from build123d import *

# Parameters (mm, degrees)
SKETCH_1_R               = 16.5
EXTRUDE_1_DEPTH          = 8
CUT_EXTRUDE_1_DEPTH      = 25.667792767
CUT_EXTRUDE_1_DEPTH_BACK = 25.667792767
SKETCH_4_R               = 2.5
SKETCH_4_R_2             = 1.9
SKETCH_1_3_R             = 10
EXTRUDE_2_DEPTH          = 8
SKETCH_1_4_R             = 10
EXTRUDE_3_DEPTH          = 60
EXTRUDE_START            = 14
SKETCH_5_R               = 16.5
EXTRUDE_4_DEPTH          = 14
CUT_EXTRUDE_START        = -14
SKETCH_6_R               = 2.5
SKETCH_6_R_2             = 1.9
CUT_EXTRUDE_2_DEPTH      = 14


with BuildPart() as part:
    # Sketch 1 → Extrude 1 (new body)
    with BuildSketch(Plane(origin=(0, 0, 0), x_dir=(1, 0, 0), z_dir=(0, 1, 0))):
        with Locations(Location((0, 0, 0), (0, 0, 270))):
            Circle(SKETCH_1_R)
    extrude(amount=EXTRUDE_1_DEPTH)

    # Sketch 4 → Cut-Extrude 1 (cut, two sides: drawn at the far end of the back side and taken through both)
    with BuildSketch(Plane(origin=(0, 8, 0), x_dir=(1, 0, 0), z_dir=(0, 1, 0)).offset(-CUT_EXTRUDE_1_DEPTH_BACK)):
        with Locations(Location((0, 10.2, 0), (0, 0, 270))):
            Circle(SKETCH_4_R)
        with Locations(Location((-6.25, 10.825317547, 0), (0, 0, 270))):
            Circle(SKETCH_4_R_2)
        with Locations(Location((6.25, 10.825317547, 0), (0, 0, 270))):
            Circle(SKETCH_4_R_2)
        with Locations(Location((12.5, 0, 0), (0, 0, 270))):
            Circle(SKETCH_4_R_2)
        with Locations(Location((6.25, -10.825317547, 0), (0, 0, 270))):
            Circle(SKETCH_4_R_2)
        with Locations(Location((-6.25, -10.825317547, 0), (0, 0, 270))):
            Circle(SKETCH_4_R_2)
        with Locations(Location((-12.5, 0, 0), (0, 0, 270))):
            Circle(SKETCH_4_R_2)
        with Locations(Location((8.833459119, -5.1, 0), (0, 0, 270))):
            Circle(SKETCH_4_R)
        with Locations(Location((-8.833459119, -5.1, 0), (0, 0, 270))):
            Circle(SKETCH_4_R)
    extrude(amount=CUT_EXTRUDE_1_DEPTH + CUT_EXTRUDE_1_DEPTH_BACK, mode=Mode.SUBTRACT)

    # Sketch 1_3 → Extrude 2 (add)
    with BuildSketch(Plane(origin=(0, 0, 0), x_dir=(1, 0, 0), z_dir=(0, 1, 0))):
        with BuildLine():
            ThreePointArc((0.989109801, 16.470326706), (16.5, 0), (0.989109801, -16.470326706))
            Line((0.989109801, -16.470326706), (100, -13.5))
            ThreePointArc((100, -13.5), (113.5, 0), (100, 13.5))
            Line((100, 13.5), (0.989109801, 16.470326706))
        make_face()
        with Locations(Location((100, 0, 0), (0, 0, 270))):
            Circle(SKETCH_1_3_R, mode=Mode.SUBTRACT)
    extrude(amount=EXTRUDE_2_DEPTH)

    # Sketch 1_4 → Extrude 3 (add)
    with BuildSketch(Plane(origin=(0, 0, 0), x_dir=(1, 0, 0), z_dir=(0, 1, 0))):
        with Locations(Location((100, 0, 0), (0, 0, 270))):
            Circle(SKETCH_1_4_R)
    extrude(amount=EXTRUDE_3_DEPTH)

    # Sketch 5 → Extrude 4 (add)
    with BuildSketch(Plane.XZ.offset(EXTRUDE_START)):
        with Locations(Location((0, 0, 0), (0, 0, 270))):
            Circle(SKETCH_5_R)
    extrude(amount=-EXTRUDE_4_DEPTH)

    # Sketch 6 → Cut-Extrude 2 (cut)
    with BuildSketch(Plane.XZ.offset(14).offset(CUT_EXTRUDE_START)):
        with Locations(Location((-8.833459119, 5.1, 0), (0, 0, 90))):
            Circle(SKETCH_6_R)
        with Locations(Location((-12.5, 0, 0), (0, 0, 90))):
            Circle(SKETCH_6_R_2)
        with Locations(Location((-6.25, -10.825317547, 0), (0, 0, 90))):
            Circle(SKETCH_6_R_2)
        with Locations(Location((0, -10.2, 0), (0, 0, 90))):
            Circle(SKETCH_6_R)
        with Locations(Location((6.25, -10.825317547, 0), (0, 0, 90))):
            Circle(SKETCH_6_R_2)
        with Locations(Location((12.5, 0, 0), (0, 0, 90))):
            Circle(SKETCH_6_R_2)
        with Locations(Location((8.833459119, 5.1, 0), (0, 0, 90))):
            Circle(SKETCH_6_R)
        with Locations(Location((6.25, 10.825317547, 0), (0, 0, 90))):
            Circle(SKETCH_6_R_2)
        with Locations(Location((-6.25, 10.825317547, 0), (0, 0, 90))):
            Circle(SKETCH_6_R_2)
    extrude(amount=CUT_EXTRUDE_2_DEPTH, mode=Mode.SUBTRACT)


solid = part.part
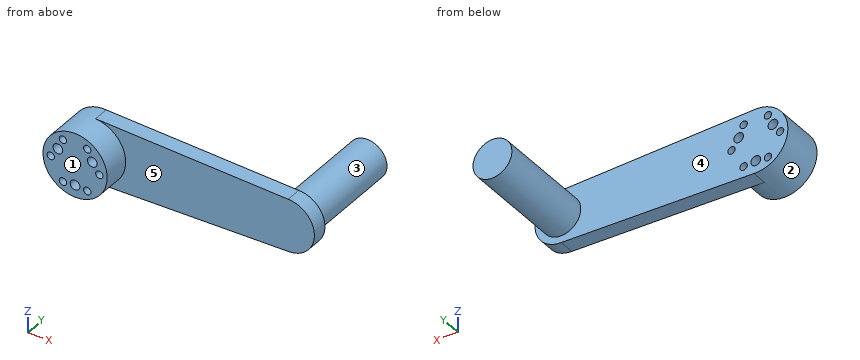
Part model, mm, in its own coordinate system. Face numbers are marked on the shaded views. A direction names the side the tool comes from. Coordinates: 2 decimals unless noted, no trailing zeros. Order: outer loops, then holes, each group sorted by start corner. A loop starts at its lowest first (then second) coordinate and runs counter-clockwise, first axis right, second up.
(1) Pull direction Y, two halves, no side cores. Call the marked faces 3, 4 and 5: pulls with the +Y half, pulls with the -Y half, needs draft (parallel to the pull), parting line crosses it, or undercut.
Check sheet entries:
face 3: needs draft
face 4: pulls with the +Y half
face 5: pulls with the -Y half
(2) Tool access for the marked faces 1 and 2: list every direction of +Z, -Z, +X, -X, +Y, -Y with a clear straight run to the whole face (end or side of a thin tool).
Check sheet entries:
face 1: +Z, -Z, +X, -X, -Y
face 2: -Y
(3) Pin check, flat tips, straight feed: pin 1 Ø16.5 at (x, z) = (47.5, 3.5) entering from -Y; pin 2 Ø6 at (x, z) = (8.83, 5.1) entering from +Y; pin 3 Ø2 at (y, z) = (25.5, -4.5) entering from +X; pin 4 Ø4.5 at (x, z) = (6.25, -10.83) entering from -Y. Stop position of each tip, or through.
Check sheet entries:
pin 1: stops at y = 0
pin 2: stops at y = 8
pin 3: stops at x = 109.37
pin 4: stops at y = -14
(4) Probe L1, parallel to X at y = -2, z = 0; L2, parallel to X at y = 0.25, z = -10.2; L3, parallel to Z at x = -6.25, y = -7.25. List the from-to ranges inside material, lowest first.
Check sheet entries:
L1: x = -16.5 to -14.4, -10.6 to 10.6, 14.4 to 16.5
L2: x = -12.97 to -8.04, -4.46 to -2.5, 2.5 to 4.46, 8.04 to 108.84
L3: z = -15.27 to -12.73, -8.93 to 8.93, 12.73 to 15.27
(5) Slice it at C-C, the plane y = 14. Write the cut outline in (x, z).
Check sheet entries:
outline: circle Ø20 at (100, 0)
(6) Slice it at D-D, the plane x = 97. Write the cut outline in (y, z), and give its area (3 significant figures).
Check sheet entries:
outline: (0, -13.59) - (8, -13.59) - (8, -9.54) - (60, -9.54) - (60, 9.54) - (8, 9.54) - (8, 13.59) - (0, 13.59) - close
area: 1,210 mm2
(7) Slice it at A-A, the plane z = 0. Write the cut outline in (x, y).
Check sheet entries:
outline: (-16.5, -14) - (-14.4, -14) - (-14.4, 8) - (-16.5, 8) - close; (-10.6, -14) - (10.6, -14) - (10.6, 8) - (-10.6, 8) - close; (14.4, -14) - (16.5, -14) - (16.5, 0) - (113.5, 0) - (113.5, 8) - (110, 8) - (110, 60) - (90, 60) - (90, 8) - (14.4, 8) - close
(8) Slice it at B-B, the plane y = -5. State how many separate pieces and enclosed holes the cut face has, and give its area (3 significant figures).
Check sheet entries:
separate pieces: 1
enclosed holes: 9
area: 728 mm2
